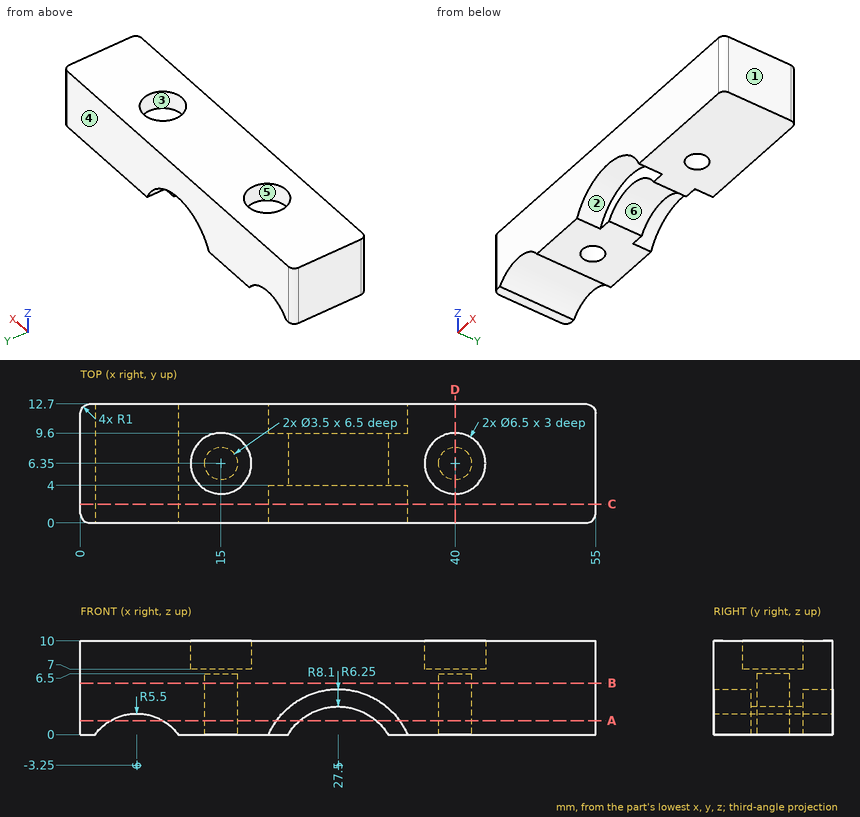
Design review of the part shown in the three views and the two pictorial views. Dimensions are in mm from the part's minimum x, y and z. A direction names the side the tool comes from. Give positions to 0.01 mm unless a question says otherwise; leave off trailing zeros. Loops run counter-clockwise (first coordinate to the right, second up) from the corner with the lowest first, then second, coordinate; pieces in that order, holes last. Notation, with made-up numbers: (1.5, -39.5) -> (34.5, -39.5) arc R26 cw to (34.5, -6.5) -> close; hole circle Ø5 at (-30.75, -5). An arc over 180 degrees is marked (long way). Answer as a JSON object with one key per item and string values. Group by question number.
Q1. Take a section at C-C (y = 2). Write out the cut boundary in (x, z), plus the area to 3 significant figures.
Q2. Insertion check: pin 1 (3 mm diameter, centred on x = 15, y = 6.35, fed in from -Z); pin 2 (5.5 mm diameter, centred on x = 40, y = 6.35, fed in from +Z). Each pin has a flat end and moves straight along its axis. Give the tip position at first contact, or say it passes through.
Q3. Take a section at B-B (z = 5.5). Write out the cut boundary in (x, y), plus the area to 3 significant figures.
Q4. Wall thickness on line 1 along Y through (x, z) = (15, 3); line 2 along X through (y, z) = (8.5, 1.25); line 3 along X through (y, z) = (7.5, 8.5): over which ranges is each line inside the solid? List them lowest first.
Q5. Take a section at D-D (x = 40). Write out the cut boundary in (y, z), plus the area to 4 significant figures.
Q6. Draft analysis for pull direction Y (two halves, no side actions). For the marked faces 4, 5 and 6, state which applies: pulls with the +Y half, pulls with the -Y half, needs draft (parallel to the pull), parting line crosses it, or undercut.
Q7. Take a section at A-A (z = 1.5). Write out the cut boundary in (x, y), plus the area to 3 significant figures.
Q8. Tool access review of the marked faces 1, 2 and 3: name each direction out of +Z, -Z, +X, -X, +Y, -Y from which nothing blocks a thin tool from reaching the whole face with its end or side.
Answer below:
{
 "1": {"outline": "(0, 0) -> (1.56, 0) arc R5.5 cw to (10.44, 0) -> (20.08, 0) arc R8.1 cw to (34.92, 0) -> (55, 0) -> (55, 10) -> (0, 10) -> close", "area": "484 mm2"},
 "2": {"pin 1": "stops at z = 6.5", "pin 2": "stops at z = 7"},
 "3": {"outline": "(0, 1) arc R1 ccw to (1, 0) -> (54, 0) arc R1 ccw to (55, 1) -> (55, 11.7) arc R1 ccw to (54, 12.7) -> (1, 12.7) arc R1 ccw to (0, 11.7) -> close; hole circle Ø3.5 at (15, 6.35); hole circle Ø3.5 at (40, 6.35)", "area": "678 mm2"},
 "4": {"line 1": "y = 0 to 4.6, 8.1 to 12.7", "line 2": "x = 0 to 2.84, 9.16 to 23.16, 31.84 to 55", "line 3": "x = 0 to 11.96, 18.04 to 36.96, 43.04 to 55"},
 "5": {"outline": "(0, 0) -> (4.6, 0) -> (4.6, 6.5) -> (8.1, 6.5) -> (8.1, 0) -> (12.7, 0) -> (12.7, 10) -> (9.6, 10) -> (9.6, 7) -> (3.1, 7) -> (3.1, 10) -> (0, 10) -> close", "area": "84.75 mm2"},
 "6": {"face 4": "pulls with the +Y half", "face 5": "undercut", "face 6": "needs draft"},
 "7": {"outline": "(0, 1) arc R1 ccw to (1, 0) -> (3.23, 0) -> (3.23, 12.7) -> (1, 12.7) arc R1 ccw to (0, 11.7) -> close; (8.77, 0) -> (20.94, 0) -> (20.94, 4) -> (23.44, 4) -> (23.44, 9.6) -> (20.94, 9.6) -> (20.94, 12.7) -> (8.77, 12.7) -> close; (31.56, 4) -> (34.06, 4) -> (34.06, 0) -> (54, 0) arc R1 ccw to (55, 1) -> (55, 11.7) arc R1 ccw to (54, 12.7) -> (34.06, 12.7) -> (34.06, 9.6) -> (31.56, 9.6) -> close; hole circle Ø3.5 at (15, 6.35); hole circle Ø3.5 at (40, 6.35)", "area": "469 mm2"},
 "8": {"face 1": "+Z, -Z, +X, +Y, -Y", "face 2": "-Z, -Y", "face 3": "+Z"}
}
